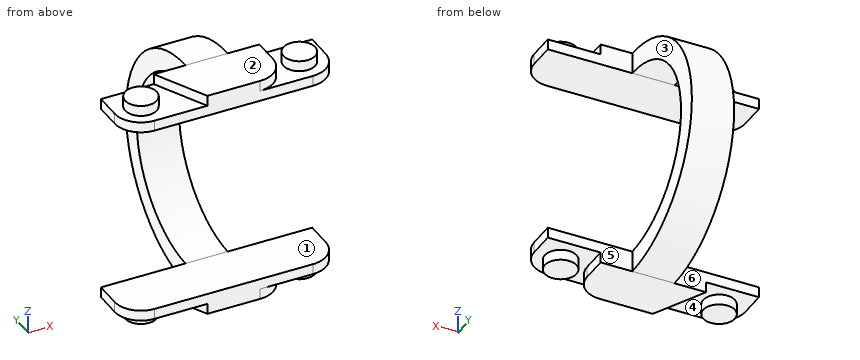
```python
from build123d import *

# Parameters (mm, degrees)
SKETCH3_W             = 2
SKETCH3_H             = 5
BOSS_EXTRUDE1_DEPTH   = 20
BOSS_EXTRUDE1_2_DEPTH = 20
SKETCH4_W             = 5
SKETCH4_H             = 5
CUT_EXTRUDE1_DEPTH    = 1
SKETCH5_W             = 5
SKETCH5_H             = 5
CUT_EXTRUDE2_DEPTH    = 1
SWEEP1_START          = 8
SWEEP1_DEPTH          = 4
SKETCH7_R             = 1.5
BOSS_EXTRUDE2_DEPTH   = 1
BOSS_EXTRUDE3_START   = 1
SKETCH8_R             = 1.5
BOSS_EXTRUDE3_DEPTH   = 1
FILLET1_R             = 2.5
CUT_EXTRUDE3_DEPTH    = 1
CUT_EXTRUDE4_DEPTH    = 1
FILLET2_R             = 2.5


# Read off the part's stored shape, not the designer's step: Sweep1
with BuildPart() as part:
    # Sketch3 → Boss-Extrude1 (new body)
    with BuildSketch(Plane(origin=(0, 0, 0), x_dir=(0, 0, -1), z_dir=(1, 0, 0))):
        with Locations((-10, 0)):
            Rectangle(SKETCH3_W, SKETCH3_H)
    extrude(amount=BOSS_EXTRUDE1_DEPTH)

    # Sketch4 → Cut-Extrude1 (cut)
    with BuildSketch(Plane.XY.offset(11)):
        with Locations((2.5, 0)):
            Rectangle(SKETCH4_W, SKETCH4_H)
        with Locations((17.5, 0)):
            Rectangle(SKETCH4_W, SKETCH4_H)
    extrude(amount=-CUT_EXTRUDE1_DEPTH, mode=Mode.SUBTRACT)



with BuildPart() as body_2:
    # Sketch3 → Boss-Extrude1 2 (new body)
    with BuildSketch(Plane(origin=(0, 0, 0), x_dir=(0, 0, -1), z_dir=(1, 0, 0))):
        with Locations((10, 0)):
            Rectangle(SKETCH3_W, SKETCH3_H)
    extrude(amount=BOSS_EXTRUDE1_2_DEPTH)

    # Sketch5 → Cut-Extrude2 (cut)
    with BuildSketch(Plane(origin=(0, 0, -11), x_dir=(-1, 0, 0), z_dir=(0, 0, -1))):
        with Locations((-17.5, 0)):
            Rectangle(SKETCH5_W, SKETCH5_H)
        with Locations((-2.5, 0)):
            Rectangle(SKETCH5_W, SKETCH5_H)
    extrude(amount=-CUT_EXTRUDE2_DEPTH, mode=Mode.SUBTRACT)


with BuildPart() as part_1:
    add(part.part)

    add(body_2.part)  # Sweep1 merges body 2
    # Sweep1 outline → Sweep1 (add)
    with BuildSketch(Plane.YZ.offset(SWEEP1_START)):
        with BuildLine():
            Line((2.5, -9), (2.5, -11))
            ThreePointArc((2.5, -11), (13.5, 0), (2.5, 11))
            Line((2.5, 11), (2.5, 9))
            ThreePointArc((2.5, 9), (11.5, 0), (2.5, -9))
        make_face()
    extrude(amount=SWEEP1_DEPTH)

    # Sketch7 → Boss-Extrude2 (add)
    with BuildSketch(Plane(origin=(0, 0, -10), x_dir=(-1, 0, 0), z_dir=(0, 0, -1))):
        with Locations(Location((-2.5, 0, 0), (0, 0, 270))):
            Circle(SKETCH7_R)
        with Locations(Location((-17.5, 0, 0), (0, 0, 90))):
            Circle(SKETCH7_R)
    extrude(amount=BOSS_EXTRUDE2_DEPTH)

    # Sketch8 → Boss-Extrude3 (add)
    with BuildSketch(Plane.XY.offset(10).offset(BOSS_EXTRUDE3_START)):
        with Locations(Location((17.5, 0, 0), (0, 0, 90))):
            Circle(SKETCH8_R)
        with Locations(Location((2.5, 0, 0), (0, 0, 270))):
            Circle(SKETCH8_R)
    extrude(amount=-BOSS_EXTRUDE3_DEPTH)

    # Fillet1
    fillet1_edges = [part_1.edges().sort_by_distance(p)[0] for p in [
        (0, -2.5, 9.5),
        (20, -2.5, 9.5),
        (20, -2.5, -9.5),
        (0, -2.5, -9.5),
    ]]
    fillet(fillet1_edges, radius=FILLET1_R)

    # Sketch9 → Cut-Extrude3 (cut)
    with BuildSketch(Plane.XY.offset(11)):
        Polygon((5, 2.5), (7.5, -2.5), (5, -2.5), align=None)
    extrude(amount=-CUT_EXTRUDE3_DEPTH, mode=Mode.SUBTRACT)

    # Sketch10 → Cut-Extrude4 (cut)
    with BuildSketch(Plane(origin=(0, 0, -11), x_dir=(-1, 0, 0), z_dir=(0, 0, -1))):
        Polygon((-5, 2.5), (-7.5, -2.5), (-5, -2.5), align=None)
    extrude(amount=-CUT_EXTRUDE4_DEPTH, mode=Mode.SUBTRACT)

    # Fillet2
    fillet2_edges = [part_1.edges().sort_by_distance(p)[0] for p in [
        (15, -2.5, 10.5),
        (15, -2.5, -10.5),
    ]]
    fillet(fillet2_edges, radius=FILLET2_R)


solid = part_1.part
```
The model under review builds one solid part; all positions refer to its coordinate system, in mm. Face numbers are marked on the shaded views. A direction names the side the tool comes from. Round coordinates to 2 decimals unless told otherwise and drop trailing zeros. Order: outer loops, then holes, each group sorted by start corner. A loop starts at its lowest first (then second) coordinate and runs counter-clockwise, first axis right, second up. Notation, with made-up numbers: (0, -15) - (8, -15) arc R3 cw to (8, -11) - close; hole circle Ø11 at (37, 72.5). An arc over 180 degrees is marked (long way). Answer in a Markdown table with one row per item.
(1) Take a section at B-B on x = 18.5. Write out the cut boundary in (y, z).
Result set:
| item | result |
|---|---|
| outline | (-2.29, -10) - (-1.12, -10) - (-1.12, -11) - (1.12, -11) - (1.12, -10) - (2.5, -10) - (2.5, -9) - (-2.29, -9) - close; (-2.29, 9) - (2.5, 9) - (2.5, 10) - (1.12, 10) - (1.12, 11) - (-1.12, 11) - (-1.12, 10) - (-2.29, 10) - close |
(2) Take a section at A-A on y = 2. Write out the cut boundary in (x, z), plus the area to 3 significant figures.
Result set:
| item | result |
|---|---|
| outline | (0, -10) - (5.25, -10) - (5.25, -11) - (15, -11) - (15, -10) - (20, -10) - (20, -9) - (0, -9) - close; (0, 9) - (20, 9) - (20, 10) - (15, 10) - (15, 11) - (5.25, 11) - (5.25, 10) - (0, 10) - close |
| area | 59.5 mm2 |
(3) Take a section at D-D on z = 0. Write out the cut boundary in (x, y), plus the area to 3 significant figures.
Result set:
| item | result |
|---|---|
| outline | (8, 11.5) - (12, 11.5) - (12, 13.5) - (8, 13.5) - close |
| area | 8.00 mm2 |
(4) Mouldability with a two-part tool opening along Z and no side actions: class the marked faces 1, 2 and 3 as released by +Z, released by -Z, zero draft, split by the parting line, or undercut.
Result set:
| item | result |
|---|---|
| face 1 | undercut |
| face 2 | released by +Z |
| face 3 | zero draft |
(5) Machinability: for the marked faces 4, 5 and 6, which of the approach directions +Z, -Z, +X, -X, +Y, -Y give a long, thin tool a straight path to every point of the face, cutting with its end or side? Answer none if there is none.
Result set:
| item | result |
|---|---|
| face 4 | -Z |
| face 5 | +Z, -Z, +X, +Y |
| face 6 | +Z, -Z, -X, +Y |
(6) Clearance check with flat-ended pins moving along their axes: P1, Ø10, axis at x = 18, z = 4.5, coming from the +Y side; P2, Ø3.5, axis at y = 10, z = 2.5, coming from the -X side; P3, Ø0.5, axis at y = 1.5, z = 10.5, coming from the +X side; P4, Ø4, axis at x = 15, y = -0.5, coming from the -Z side. State where each tip first meets the part, or that it passes through.
Result set:
| item | result |
|---|---|
| P1 | stops at y = 2.5 |
| P2 | stops at x = 8 |
| P3 | stops at x = 18.33 |
| P4 | stops at z = -11 |
(7) Take a section at C-C on x = 11.5. Write out the cut boundary in (y, z).
Result set:
| item | result |
|---|---|
| outline | (-2.5, -11) - (2.5, -11) arc R11 ccw to (2.5, 11) - (-2.5, 11) - (-2.5, 9) - (2.5, 9) arc R9 cw to (2.5, -9) - (-2.5, -9) - close |
(8) For line 1 (Z direction, x = 15.25, y = -1.75); line 2 (Z direction, x = 18.5, y = -1); line 3 (Y direction, x = 11.5, z = 1), list the stretches that pass through material, from the lowest coordinate up. Write a range as from..to.
Result set:
| item | result |
|---|---|
| line 1 | z = -10..-9, 9..10 |
| line 2 | z = -11..-9, 9..11 |
| line 3 | y = 11.44..13.45 |
